Check sheet for the drawn part. Datum: minimum x, y, z corner. Units: mm. Coordinates: 2 decimals unless noted, no trailing zeros. Order: outer loops, then holes, each group sorted by start corner. A loop starts at its lowest first (then second) coordinate and runs counter-clockwise, first axis right, second up.
1. Cross-section at B-B (x = 7). Enter the section's corners in (y, z).
2. Gauge pin test, flat ends, axial feed: pin 1 Ø2 at (x, y) = (87.5, 2) entering from -Z; pin 2 Ø1.2 at (x, y) = (19.5, 1.5) entering from +Z; pin 3 Ø2 at (x, y) = (88, 2.5) entering from +Z; pin 4 Ø1.5 at (y, z) = (0.5, 54) entering from -X. Record the tip position at first contact, or that the pin passes through.
3. Cross-section at A-A (y = 2.25). Enter the section's corners in (x, z), then the cut area to 3 significant figures.
4. Cross-section at C-C (z = 72). Enter the section's corners in (x, y).
5. Thickness scan on line 1 (Z direction, x = 64.5, y = 0.85); line 2 (X direction, y = 0.25, z = 228). Record the ranges inside material, lowest first.
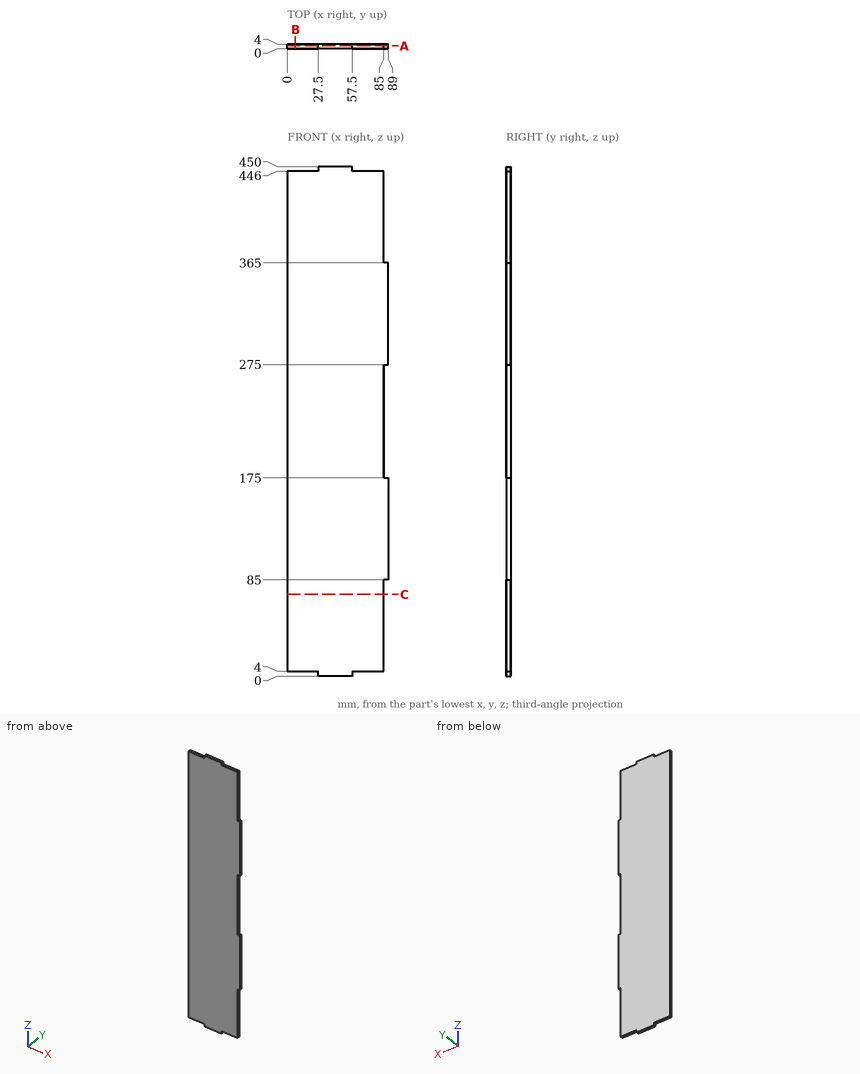
Data:
1. outline: (0, 4) - (4, 4) - (4, 446) - (0, 446) - close
2. pin 1: stops at z = 85
2. pin 2: stops at z = 446
2. pin 3: stops at z = 365
2. pin 4: stops at x = 0
3. outline: (0, 4) - (27.5, 4) - (27.5, 0) - (57.5, 0) - (57.5, 4) - (85, 4) - (85, 85) - (89, 85) - (89, 175) - (85, 175) - (85, 275) - (89, 275) - (89, 365) - (85, 365) - (85, 446) - (57.5, 446) - (57.5, 450) - (27.5, 450) - (27.5, 446) - (0, 446) - close
3. area: 38,500 mm2
4. outline: (0, 0) - (85, 0) - (85, 4) - (0, 4) - close
5. line 1: z = 4 to 446
5. line 2: x = 0 to 85
